Check sheet for the modelled part. Datum: model origin and axes. Units: mm. Face numbers are marked on the shaded views. A direction names the side the tool comes from. Round coordinates to 2 decimals unless told otherwise and drop trailing zeros. Write each loop counter-clockwise with the first axis right and the second up, starting at its lowest first coordinate (ties: lowest second). Pieces come first, ordered by that corner, then holes. Notation, with made-up numbers: M 86.5,56 L 126.5,56 A25 cw 126.5,70 Z; hole C 5,27 d2. An arc over 180 degrees is marked long. Put each result on its own line as item: value.
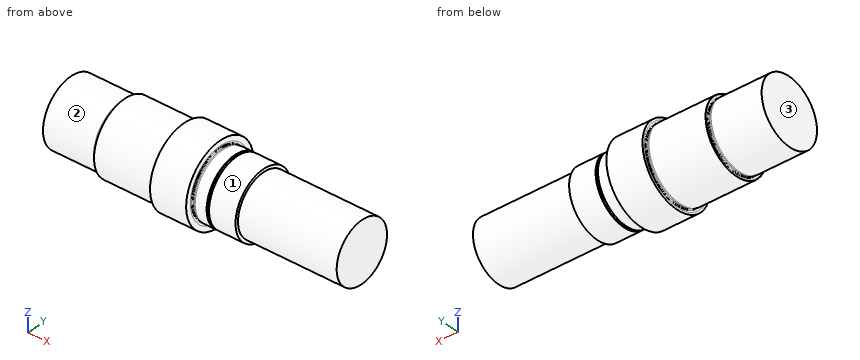
```python
from build123d import *


with BuildPart() as part:
    # Skizze1 → Rotation1 (revolve)
    with BuildSketch(Plane(origin=(0, 0, 0), x_dir=(1, 0, 0), z_dir=(0, 1, 0))):
        with BuildLine():
            Line((0, 0), (0, 27.5))
            Line((0, 27.5), (42, 27.5))
            Line((42, 27.5), (43.043315314, 27.220444504))
            ThreePointArc((43.043315314, 27.220444504), (43.120291025, 27.205133083), (43.198606741, 27.2))
            Line((43.198606741, 27.2), (44.067315551, 27.2))
            ThreePointArc((44.067315551, 27.2), (44.544808566, 27.417606104), (44.693842758, 27.920737106))
            Line((44.693842758, 27.920737106), (44.5, 29.3))
            Line((44.5, 29.3), (44.5, 30))
            Line((44.5, 30), (91.5, 30))
            Line((91.5, 30), (92.543315314, 29.720444504))
            ThreePointArc((92.543315314, 29.720444504), (92.620291025, 29.705133083), (92.698606741, 29.7))
            Line((92.698606741, 29.7), (93.6, 29.7))
            ThreePointArc((93.6, 29.7), (94.052155597, 29.905594985), (94.19444145, 30.38148228))
            Line((94.19444145, 30.38148228), (94, 31.8))
            Line((94, 31.8), (94, 33.5))
            Line((94, 33.5), (124, 33.5))
            Line((124, 33.5), (124, 29.3))
            Line((124, 29.3), (123.80555855, 27.88148228))
            ThreePointArc((123.80555855, 27.88148228), (123.947844403, 27.405594985), (124.4, 27.2))
            Line((124.4, 27.2), (125.301393259, 27.2))
            ThreePointArc((125.301393259, 27.2), (125.379708975, 27.205133083), (125.456684686, 27.220444504))
            Line((125.456684686, 27.220444504), (126.5, 27.5))
            Line((126.5, 27.5), (136, 27.5))
            Line((136, 27.5), (136, 26.5))
            Line((136, 26.5), (138, 26.5))
            Line((138, 26.5), (138, 27.5))
            Line((138, 27.5), (160, 27.5))
            Line((160, 27.5), (160, 25))
            Line((160, 25), (242, 25))
            Line((242, 25), (242, 0))
            Line((242, 0), (0, 0))
        make_face()
    revolve(axis=Axis((242, 0, 0), (-1, 0, 0)))


solid = part.part
```
1. Scan lines: probe 1 along X at (y, z) = (22.5, -15); probe 2 along Y at (x, z) = (54, -1); probe 3 along Y at (x, z) = (38.5, -11.5). Record each from-to range of solid material in increasing order.
Computed values:
probe 1: x = 0 to 136, 138 to 160
probe 2: y = -29.98 to 29.98
probe 3: y = -24.98 to 24.98
2. Access from +Z, -Z, +X, -X, +Y, -Y to the whole of each face (thin tool, end or side, straight path). Record for the marked faces 1, 2 and 3.
Computed values:
face 1: +X
face 2: -X
face 3: +Z, -Z, -X, +Y, -Y
3. Cross-section at A-A (x = 78.5). Enter the section's corners in (y, z).
Computed values:
outline: C 0,0 d60
4. Cross-section at B-B (x = 17). Enter the section's corners in (y, z).
Computed values:
outline: C 0,0 d55
5. Depth check by flat-ended pin: pin 1 Ø1 at (x, y) = (178.5, -9) entering from +Z; pin 2 Ø12 at (x, y) = (217, 21.5) entering from +Z; pin 3 Ø3 at (x, z) = (154.5, 11) entering from -Y. Enter the tip coordinate at first touch or a pass-through.
Computed values:
pin 1: stops at z = 23.51
pin 2: stops at z = 19.62
pin 3: stops at y = -25.81
